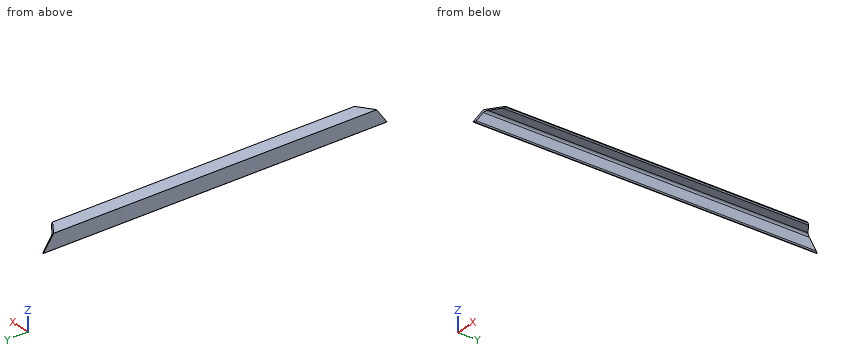
from build123d import *

# Parameters (mm, degrees)
F1_DEPTH  = 1154
F7_DEPTH  = 45
F9_DEPTH  = 45
F11_W     = 4.8190290108
F11_H     = 1158.3167838398
F12_DEPTH = 0.5


with BuildPart() as f1:
    # F0 (on Front) → F1 (new body)
    with BuildSketch(Plane.XZ):
        with BuildLine():
            Line((-9.4517558242, 28.4011573891), (-9.4517558242, -21.5988426109))
            Line((-9.4517558242, -21.5988426109), (-6.9517558242, -21.5988426109))
            ThreePointArc((-6.9517558242, -21.5988426109), (-4.47688209, -20.5737163451), (-3.4517558242, -18.0988426109))
            Line((-3.4517558242, -18.0988426109), (-3.4517558242, 15.4011573891))
            ThreePointArc((-3.4517558242, 15.4011573891), (-1.4015032925, 20.3509048574), (3.5482441758, 22.4011573891))
            Line((3.5482441758, 22.4011573891), (37.0482441758, 22.4011573891))
            ThreePointArc((37.0482441758, 22.4011573891), (39.52311791, 23.4262836549), (40.5482441758, 25.9011573891))
            Line((40.5482441758, 25.9011573891), (40.5482441758, 28.4011573891))
            Line((40.5482441758, 28.4011573891), (-9.4517558242, 28.4011573891))
        make_face()
    extrude(amount=F1_DEPTH)

    # F6 (on 3pt) → F7 (cut)
    with BuildSketch(Plane(origin=(8.0484171275, 0, -8.0484171275), x_dir=(0, -1, 0), z_dir=(-0.7071067812, 0, 0.7071067812))):
        Polygon((0, 48.7545894053), (0, -21.9560887134), (70.7106781187, 48.7545894053), align=None)
    extrude(amount=F7_DEPTH, mode=Mode.SUBTRACT)

    # F8 (on 3pt) → F9 (cut)
    with BuildSketch(Plane(origin=(8.0484171275, 0, -8.0484171275), x_dir=(0, -1, 0), z_dir=(-0.7071067812, 0, 0.7071067812))):
        Polygon((1083.2893218813, 48.7545894053), (1154, -21.9560887134), (1154, 48.7545894053), align=None)
    extrude(amount=F9_DEPTH, mode=Mode.SUBTRACT)

    # F11 (on face) → F12 (cut)
    with BuildSketch(Plane(origin=(-15.5252992176, 0, -15.5252992176), x_dir=(0.7071067812, 0, -0.7071067812), z_dir=(-0.7071067812, 0, -0.7071067812))):
        with Locations((8.6135719903, 577.1591997473)):
            Rectangle(F11_W, F11_H)
    extrude(amount=-F12_DEPTH, mode=Mode.SUBTRACT)


solid = f1.part
The listing builds one solid part. Answer for the finished solid, in the listing's coordinates (mm). Coordinates: 2 decimals unless noted, no trailing zeros. Order: outer loops, then holes, each group sorted by start corner. A loop starts at its lowest first (then second) coordinate and runs counter-clockwise, first axis right, second up.
Q1. Given P1, Ø2, axis at y = -801, z = 1.5, coming from the +X side; P2, Ø1, axis at x = 9, z = 21.5, coming from the -Y side; P3, Ø17, axis at x = 12.5, y = -395.5, coming from the -Z side, each flat-ended and moving along its own axis, determine where each tip first touches the part or whether it passes through.
Q2. A cutting plane is placed at B-B, the plane x = 13. Write down the section's boundary in (y, z).
Q3. A cutting plane is placed at A-A, the plane y = -489. Write down the section's boundary in (x, z).
Q4. A cutting plane is placed at C-C, the plane z = 1.5. Write down the section's boundary in (x, y), and give its area (3 significant figures).
Q5. Consider line 1 (Z direction, x = 15.5, y = -297.5); line 2 (X direction, y = -903.5, z = -14); line 3 (Y direction, x = -6.5, z = -14). Determine where each line is inside the solid, lowest interval first.
Answers follow:
1. P1: stops at x = -3.45
1. P2: passes through
1. P3: stops at z = 22.4
2. outline: (-1107.01, 22.4) - (-46.99, 22.4) - (-51.23, 28.4) - (-1102.77, 28.4) - close
3. outline: (-9.45, -20.89) - (-8.74, -21.6) - (-6.95, -21.6) arc R3.5 ccw to (-3.45, -18.1) - (-3.45, 15.4) arc R7 cw to (3.55, 22.4) - (37.05, 22.4) arc R3.5 ccw to (40.55, 25.9) - (40.55, 28.4) - (-9.45, 28.4) - close
4. outline: (-9.45, -1137.67) - (-3.45, -1133.42) - (-3.45, -20.58) - (-9.45, -16.33) - close
4. area: 6,700 mm2
5. line 1: z = 22.4 to 28.4
5. line 2: x = -9.45 to -3.45
5. line 3: y = -1146.54 to -7.46
